Can you work these out from the model? Positions are in its coordinate system, mm. Give positions to 0.01 mm unless a question says otherwise; leave off trailing zeros.
```python
from build123d import *

# Parameters (mm, degrees)
F0_R     = 1.524
F0_R_2   = 1.1938
F1_DEPTH = 2.9972


with BuildPart() as f1:
    # F0 (on Top) → F1 (new body)
    with BuildSketch(Plane.XY):
        with BuildLine():
            ThreePointArc((0, 3.048), (0.892739, 0.892739), (3.048, 0))
            Line((3.048, 0), (110.998, 0))
            ThreePointArc((110.998, 0), (113.153261, 0.892739), (114.046, 3.048))
            Line((114.046, 3.048), (114.046, 53.848))
            ThreePointArc((114.046, 53.848), (113.153261, 56.003261), (110.998, 56.896))
            Line((110.998, 56.896), (3.048, 56.896))
            ThreePointArc((3.048, 56.896), (0.892739, 56.003261), (0, 53.848))
            Line((0, 53.848), (0, 3.048))
        make_face()
        with Locations((3.048, 3.048)):
            Circle(F0_R, mode=Mode.SUBTRACT)
        with Locations((20.193, 4.318)):
            Circle(F0_R_2, mode=Mode.SUBTRACT)
        with Locations((72.263, 9.398)):
            Circle(F0_R_2, mode=Mode.SUBTRACT)
        with Locations((110.998, 3.048)):
            Circle(F0_R, mode=Mode.SUBTRACT)
        with Locations((102.743, 4.318)):
            Circle(F0_R_2, mode=Mode.SUBTRACT)
        with Locations((3.048, 53.848)):
            Circle(F0_R, mode=Mode.SUBTRACT)
        with Locations((21.463, 52.578)):
            Circle(F0_R_2, mode=Mode.SUBTRACT)
        with Locations((72.263, 37.338)):
            Circle(F0_R_2, mode=Mode.SUBTRACT)
        with Locations((96.393, 52.578)):
            Circle(F0_R_2, mode=Mode.SUBTRACT)
        with Locations((110.998, 53.848)):
            Circle(F0_R, mode=Mode.SUBTRACT)
    extrude(amount=F1_DEPTH)


solid = f1.part
```
1) For pin 1 Ø1.8 at (x, y) = (110.998, 3.048) entering from -Z (3 decimals), with a flat end and sliding along its axis, tell me the tip position at first contact or that it passes through.
Values follow:
pin 1: passes through
2) If we mould it in two halves opening along X, with no side actions, what happens to faces 1 (the face through (56, 0, 1)), 2 (the face through (19.31, 5.12, 1.48)), 3 (the face through (0.869, 0.917, 1.478)), 4 (the face through (113.13, 0.87, 1.48))? For each: +X half, -X half, draft (parallel to the pull), parting line (faces both ways), or undercut.
Values follow:
face 1: draft
face 2: undercut
face 3: -X half
face 4: +X half
3) Please list where these lines run through material, in increasing order: L1, parallel to X at y = 37.5, z = 2.3; L2, parallel to X at y = 52.5, z = 0.7; L3, parallel to X at y = 10, z = 2.15.
Values follow:
L1: x = 0 to 71.08, 73.45 to 114.05
L2: x = 0 to 2.34, 3.76 to 20.27, 22.65 to 95.2, 97.58 to 110.29, 111.71 to 114.05
L3: x = 0 to 71.23, 73.29 to 114.05
